For this review, use the dimensioned drawing (mm, ordinates from the lowest corner) and the shaded views. A direction names the side the tool comes from. Coordinates: 2 decimals unless noted, no trailing zeros. Write each loop counter-clockwise with the first axis right and the second up, starting at its lowest first coordinate (ties: lowest second). Pieces come first, ordered by that corner, then holes. Notation, with made-up numbers: M 84,34.25 L 120,34.25 A32 ccw 120,64.25 Z; hole C 76,44.5 d1. An arc over 180 degrees is marked long. Return JSON: item names as keys, results as strings.
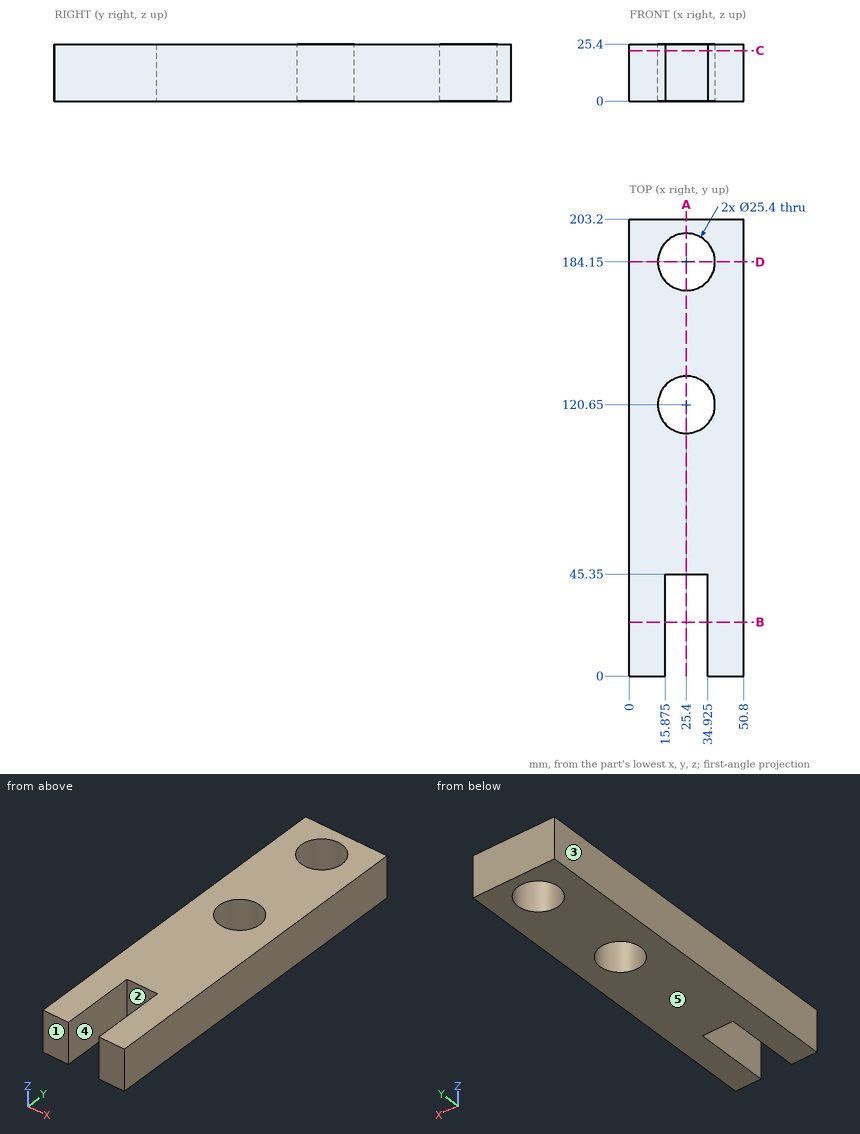
1. Draft analysis for pull direction X (two halves, no side actions). For the marked faces 3, 4 and 5, state which applies: +X half, -X half, draft (parallel to the pull), parting line (faces both ways), or undercut.
Checks:
{"face 3": "-X half", "face 4": "undercut", "face 5": "draft"}
2. Clearance check with flat-ended pins moving along their axes: pin 1 Ø1.5 at (x, z) = (7.5, 4) entering from -Y; pin 2 Ø20.5 at (x, y) = (25.4, 184.15) entering from +Z; pin 3 Ø3 at (x, z) = (32.5, 15) entering from -Y. State where each tip first meets the part, or that it passes through.
Checks:
{"pin 1": "y = 0", "pin 2": "through", "pin 3": "y = 45.35"}
3. We need section D-D (y = 184.15). State the section outline as (x, z) points.
Checks:
{"outline": "M 0,0 L 12.7,0 L 12.7,25.4 L 0,25.4 Z; M 38.1,0 L 50.8,0 L 50.8,25.4 L 38.1,25.4 Z"}
4. For the marked faces 1 and 2, list the 3-axis set-ups (+Z, -Z, +X, -X, +Y, -Y) from which the entire face can be reached by the end or side of a thin tool; tool diameter is ignored.
Checks:
{"face 1": "+Z, -Z, +X, -X, -Y", "face 2": "+Z, -Z, -Y"}
5. We need section B-B (y = 24). State the section outline as (x, z) points (3 decimals).
Checks:
{"outline": "M 0,0 L 15.875,0 L 15.875,25.4 L 0,25.4 Z; M 34.925,0 L 50.8,0 L 50.8,25.4 L 34.925,25.4 Z"}
6. Wall thickness on L1, parallel to Y at x = 25.4, z = 9; L2, parallel to X at y = 32.5, z = 15.5 (3 decimals); L3, parallel to Y at x = 15.5, z = 20.5 (1 decimal): over which ranges is each line inside the solid? List them lowest first. Write a range as from..to.
Checks:
{"L1": "45.35..107.95, 133.35..171.45, 196.85..203.2", "L2": "0..15.875, 34.925..50.8", "L3": "0..112.7, 128.6..176.2, 192.1..203.2"}
7. We need section C-C (z = 22.5). Give the number of separate pieces and of enclosed holes in the cut face.
Checks:
{"separate pieces": "1", "enclosed holes": "2"}
8. We need section A-A (x = 25.4). State the section outline as (y, z) points.
Checks:
{"outline": "M 45.35,0 L 107.95,0 L 107.95,25.4 L 45.35,25.4 Z; M 133.35,0 L 171.45,0 L 171.45,25.4 L 133.35,25.4 Z; M 196.85,0 L 203.2,0 L 203.2,25.4 L 196.85,25.4 Z"}
